Check sheet for the modelled part. Datum: model origin and axes. Units: mm. A direction names the side the tool comes from. Coordinates: 2 decimals unless noted, no trailing zeros. Loops run counter-clockwise (first coordinate to the right, second up) from the corner with the lowest first, then second, coordinate; pieces in that order, holes last. Notation, with made-up numbers: M 10,22 L 60,22 A36 ccw 60,60 Z; hole C 76,-22.5 d4. An arc over 180 degrees is marked long. Return JSON: item names as keys, results as strings.
from build123d import *

# Parameters (mm, degrees)
POCKET_DEPTH = 1


with BuildPart() as part:
    # Sketch → Revolution (revolve)
    with BuildSketch(Plane.XY):
        with BuildLine():
            Line((0, -6), (1.4, -6))
            Line((1.4, -6), (1.5, -5.9))
            Line((1.5, -5.9), (1.5, 0))
            Line((1.5, 0), (2.579564, 0))
            ThreePointArc((2.579564, 0), (2.876857, 0.123143), (3, 0.420436))
            Line((3, 1.808972), (3, 0.420436))
            ThreePointArc((3, 1.808972), (1.973047, 2.323042), (0.838329, 2.5))
            Line((0.838329, 2.5), (0, 2.5))
            Line((0, 2.5), (0, -6))
        make_face()
    revolve(axis=Axis((0, 0, 0), (0, 1, 0)))

    # Sketch001 (on Face2 of Revolution) → Pocket (cut)
    with BuildSketch(Plane(origin=(0, 2.5, 0), x_dir=(-1, 0, 0), z_dir=(0, 1, 0))):
        Polygon((-0.478807, 2), (0.478807, 2), (0.478807, 0.510631), (2, 0.510631), (2, -0.510631), (0.478807, -0.510631), (0.478807, -2), (-0.478807, -2), (-0.478807, -0.510631), (-2, -0.510631), (-2, 0.510631), (-0.478807, 0.510631), align=None)
    extrude(amount=-POCKET_DEPTH, mode=Mode.SUBTRACT)


solid = part.part
1) Draft check along Z on faces 1 (the face through (-1.5, -2.91, -0.07)), 2 (the face through (0, -6, 0)), 3 (the face through (0.479, 2, 1)). Enter one of: +Z half, -Z half, draft (parallel to the pull), parting line (faces both ways), or undercut.
Answers:
{"face 1": "parting line", "face 2": "draft", "face 3": "undercut"}
2) Scan lines: line 1 along Z through (x, y) = (2.5, 1.75); line 2 along X through (y, z) = (0.75, -0.25); line 3 along X through (y, z) = (-0.5, -0.25). Record each from-to range of solid material in increasing order. Write a range as [from, to].
Answers:
{"line 1": "[-1.66, 1.66]", "line 2": "[-2.99, 2.99]", "line 3": "[-1.48, 1.48]"}
3) Set-up check for faces 4 (the face through (0, 2, 2)), 5 (the face through (0, 0, 2)), 6 (the face through (-3, 1, 0)): record each of +Z, -Z, +X, -X, +Y, -Y from which the full face is reachable in a straight line by a thin tool's end or side.
Answers:
{"face 4": "+Y", "face 5": "-Y", "face 6": "+Y, -Y"}
4) Section check B-B on y = 1. Record the cut outline in (x, z), then the cut area to 3 significant figures.
Answers:
{"outline": "C 0,0 d6", "area": "28.3 mm²"}
5) Section check A-A on y = -3.75. Record the cut outline in (x, z).
Answers:
{"outline": "C 0,0 d3"}
6) Go/stop test with flat-tipped pins: pin 1 Ø1.5 at (y, z) = (-2, 1.5) entering from +X; pin 2 Ø0.8 at (x, y) = (-1, 2) entering from -Z; pin 3 Ø1.1 at (y, z) = (2, -1.5) entering from -X. Record where each tip stops, or that it passes through.
Answers:
{"pin 1": "x = 1.3", "pin 2": "z = -2.93", "pin 3": "x = -2.83"}
